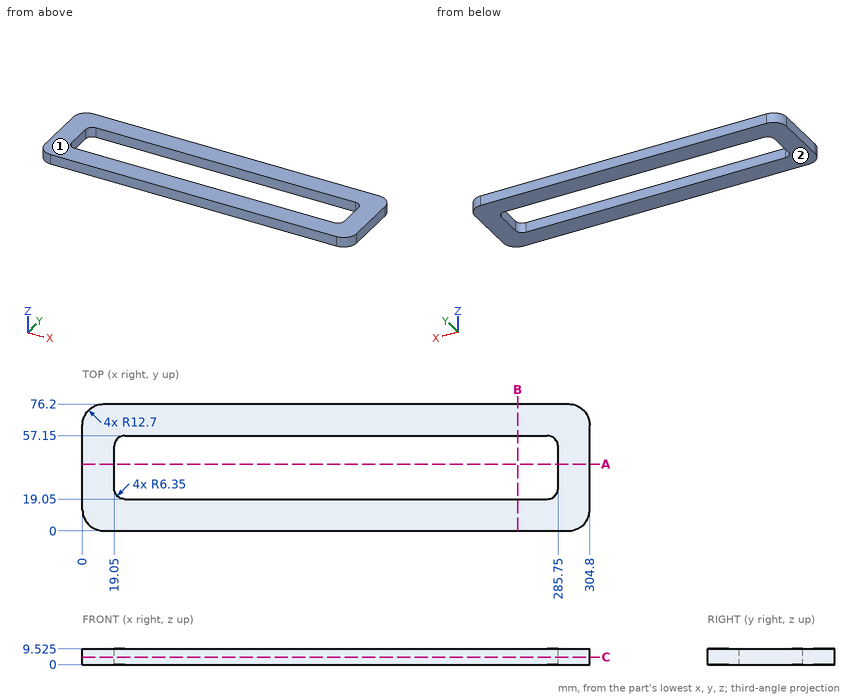
Here's the drawing with two shaded views (mm, measured from the low corner). I have some questions. Give positions to 0.01 mm unless a question says otherwise; leave off trailing zeros. Order: outer loops, then holes, each group sorted by start corner. A loop starts at its lowest first (then second) coordinate and runs counter-clockwise, first axis right, second up. Notation, with made-up numbers: M 71,78 L 126,78 A27 cw 126,100 Z; hole C 78,75.25 d1. An arc over 180 degrees is marked long. One line per question, with ' | ' between items.
Item 1: I'm going to push a flat-ended pin straight in: pin 1 Ø2 at (y, z) = (67, 2.5) entering from -X. Where does the tip first touch, or does it pass through?
Answer block:
pin 1: stops at x = 0.25
Item 2: Suppose I cut it at C-C, the plane z = 4.5. Write out the boundary of the cut face in (x, y).
Answer block:
outline: M 0,12.7 A12.7 ccw 12.7,0 L 292.1,0 A12.7 ccw 304.8,12.7 L 304.8,63.5 A12.7 ccw 292.1,76.2 L 12.7,76.2 A12.7 ccw 0,63.5 Z; hole M 19.05,25.4 A6.35 ccw 25.4,19.05 L 279.4,19.05 A6.35 ccw 285.75,25.4 L 285.75,50.8 A6.35 ccw 279.4,57.15 L 25.4,57.15 A6.35 ccw 19.05,50.8 Z
Item 3: Suppose I cut it at B-B, the plane x = 261.5. Write out the boundary of the cut face in (y, z) (3 decimals), then the cut area to 3 significant figures.
Answer block:
outline: M 0,0 L 19.05,0 L 19.05,9.525 L 0,9.525 Z; M 57.15,0 L 76.2,0 L 76.2,9.525 L 57.15,9.525 Z | area: 363 mm2
Item 4: Suppose I cut it at A-A, the plane y = 40. Write out the boundary of the cut face in (x, z) (3 decimals).
Answer block:
outline: M 0,0 L 19.05,0 L 19.05,9.525 L 0,9.525 Z; M 285.75,0 L 304.8,0 L 304.8,9.525 L 285.75,9.525 Z
Item 5: We'd pull the mould along Z, two halves only. Please class the marked faces 1 and 2: released by +Z, released by -Z, zero draft, split by the parting line, or undercut.
Answer block:
face 1: released by +Z | face 2: released by -Z
Item 6: Please list where these lines run through material, in increasing order: L1, parallel to X at y = 30.5, z = 7.75; L2, parallel to Y at x = 52.5, z = 8.5; L3, parallel to X at y = 54, z = 2.5.
Answer block:
L1: x = 0 to 19.05, 285.75 to 304.8 | L2: y = 0 to 19.05, 57.15 to 76.2 | L3: x = 0 to 19.92, 284.88 to 304.8
